The listing builds one solid part. Answer for the finished solid, in the listing's coordinates (mm). A direction names the side the tool comes from. Coordinates: 2 decimals unless noted, no trailing zeros. Loops run counter-clockwise (first coordinate to the right, second up) from the corner with the lowest first, then second, coordinate; pieces in that order, holes last. Notation, with made-up numbers: (81.5, 26) - (138.5, 26) arc R37 ccw to (138.5, 65) - close; hole circle Ø6 at (18, 62). An arc over 180 degrees is marked (long way). Return JSON: item names as keys, results as strings. Group by question number.
1. The mould has two halves that part along Y. Classify faces 1 (the face through (7, 0, 0)), 2 (the face through (-3.47, -15.62, 2.46)), 3 (the face through (10.331, 0.526, 4.341)): pulls with the +Y half, pulls with the -Y half, needs draft (parallel to the pull), parting line crosses it, or undercut.
2. Each of these flat-tipped pins is pushed along its axis until it touches: P1, Ø8, axis at y = -1, z = 17, coming from the +X side; P2, Ø5, axis at x = 12, y = 0, coming from the -Z side; P3, Ø4, axis at x = 8, z = 3.5, coming from the +Y side; P4, Ø2, axis at x = 12, y = 0, coming from the -Z side. Where does it stop, or does it pass through?
3. Section B-B (y = 0) is taken. State how many separate pieces and enclosed holes the cut face has, and give its area (3 significant figures).
4. Section A-A (z = 4.25) is taken. Write down the section's boundary in (x, y), and give its area (3 significant figures).
5. Section D-D (z = 11) is taken. Write down the section's boundary in (x, y).
6. Which of the six approach directions +Z, -Z, +X, -X, +Y, -Y give full straight-line access (tool end or side, diameter ignored) to faces 4 (the face through (0.228, -10.265, 4.341)), 5 (the face through (10.6, -1.4, 3.7)), 6 (the face through (-5.158, -3.955, 24.059))?
7. Find the intervals of material crossed by line 1 along Y through (x, z) = (0, 4.3); line 2 along Y through (x, z) = (0, 13); line 3 along Z through (x, y) = (9.5, -2.5), in increasing order.
```python
from build123d import *

# Parameters (mm, degrees)
IZIM1_R                     = 16
Y_KSEKLIK_EKSTR_ZYON1_DEPTH = 5
IZIM2_R                     = 8
Y_KSEKLIK_EKSTR_ZYON2_DEPTH = 19.7
KES_EKSTR_ZYON1_REACH       = 35.498
IZIM3_R                     = 4
KES_EKSTR_ZYON2_REACH       = 35.498
IZIM4_R                     = 1.75
IZIM4_3_R                   = 3.25
IZIM4_3_R_2                 = 1.75
KES_EKSTR_ZYON3_DEPTH       = 3.7
IZIM5_R                     = 6.5
KES_EKSTR_ZYON4_DEPTH       = 1.3
KES_EKSTR_ZYON5_START       = -23.4
IZIM5_2_R                   = 6.5
KES_EKSTR_ZYON5_DEPTH       = 1.3


with BuildPart() as part:
    # Çizim1 → Yükseklik-Ekstrüzyon1 (new body)
    with BuildSketch(Plane.XY):
        Circle(IZIM1_R)
    extrude(amount=Y_KSEKLIK_EKSTR_ZYON1_DEPTH)

    # Çizim2 → Yükseklik-Ekstrüzyon2 (add)
    with BuildSketch(Plane.XY.offset(5)):
        Circle(IZIM2_R)
    extrude(amount=Y_KSEKLIK_EKSTR_ZYON2_DEPTH)

    # Çizim3 → Kes-Ekstrüzyon1 (cut, up to next)
    with BuildSketch(Plane.XY.offset(24.7), mode=Mode.PRIVATE) as kes_ekstr_zyon1_sk1:
        Circle(IZIM3_R)
    kes_ekstr_zyon1_tool1 = extrude(kes_ekstr_zyon1_sk1.sketch, amount=-KES_EKSTR_ZYON1_REACH, mode=Mode.PRIVATE) & part.part
    add(kes_ekstr_zyon1_tool1.solids().sort_by_distance((0, 0, 24.7))[0], mode=Mode.SUBTRACT)

    # Çizim4 → Kes-Ekstrüzyon2 (cut, up to next)
    with BuildSketch(Plane(origin=(0, 0, 0), x_dir=(-1, 0, 0), z_dir=(0, 0, -1)), mode=Mode.PRIVATE) as kes_ekstr_zyon2_sk1:
        with Locations((0, 12)):
            Circle(IZIM4_R)
    kes_ekstr_zyon2_tool1 = extrude(kes_ekstr_zyon2_sk1.sketch, amount=-KES_EKSTR_ZYON2_REACH, mode=Mode.PRIVATE) & part.part
    # Çizim4 → Kes-Ekstrüzyon2 (cut, up to next)
    with BuildSketch(Plane(origin=(0, 0, 0), x_dir=(-1, 0, 0), z_dir=(0, 0, -1)), mode=Mode.PRIVATE) as kes_ekstr_zyon2_sk2:
        with Locations((12, 0)):
            Circle(IZIM4_R)
    kes_ekstr_zyon2_tool2 = extrude(kes_ekstr_zyon2_sk2.sketch, amount=-KES_EKSTR_ZYON2_REACH, mode=Mode.PRIVATE) & part.part
    # Çizim4 → Kes-Ekstrüzyon2 (cut, up to next)
    with BuildSketch(Plane(origin=(0, 0, 0), x_dir=(-1, 0, 0), z_dir=(0, 0, -1)), mode=Mode.PRIVATE) as kes_ekstr_zyon2_sk3:
        with Locations((0, -12)):
            Circle(IZIM4_R)
    kes_ekstr_zyon2_tool3 = extrude(kes_ekstr_zyon2_sk3.sketch, amount=-KES_EKSTR_ZYON2_REACH, mode=Mode.PRIVATE) & part.part
    # Çizim4 → Kes-Ekstrüzyon2 (cut, up to next)
    with BuildSketch(Plane(origin=(0, 0, 0), x_dir=(-1, 0, 0), z_dir=(0, 0, -1)), mode=Mode.PRIVATE) as kes_ekstr_zyon2_sk4:
        with Locations((-12, 0)):
            Circle(IZIM4_R)
    kes_ekstr_zyon2_tool4 = extrude(kes_ekstr_zyon2_sk4.sketch, amount=-KES_EKSTR_ZYON2_REACH, mode=Mode.PRIVATE) & part.part
    add(kes_ekstr_zyon2_tool1.solids().sort_by_distance((0, 12, 0))[0], mode=Mode.SUBTRACT)
    add(kes_ekstr_zyon2_tool2.solids().sort_by_distance((-12, 0, 0))[0], mode=Mode.SUBTRACT)
    add(kes_ekstr_zyon2_tool3.solids().sort_by_distance((0, -12, 0))[0], mode=Mode.SUBTRACT)
    add(kes_ekstr_zyon2_tool4.solids().sort_by_distance((12, 0, 0))[0], mode=Mode.SUBTRACT)

    # Çizim4<3> → Kes-Ekstrüzyon3 (cut)
    # profile 1 of 4: a face of its own
    with BuildSketch(Plane(origin=(0, 0, 0), x_dir=(-1, 0, 0), z_dir=(0, 0, -1))):
        with Locations((0, 12)):
            Circle(IZIM4_3_R)
        with Locations((0, 12)):
            Circle(IZIM4_3_R_2, mode=Mode.SUBTRACT)
    # profile 2 of 4: a face of its own
    with BuildSketch(Plane(origin=(0, 0, 0), x_dir=(-1, 0, 0), z_dir=(0, 0, -1))):
        with Locations((12, 0)):
            Circle(IZIM4_3_R)
        with Locations((12, 0)):
            Circle(IZIM4_3_R_2, mode=Mode.SUBTRACT)
    # profile 3 of 4: a face of its own
    with BuildSketch(Plane(origin=(0, 0, 0), x_dir=(-1, 0, 0), z_dir=(0, 0, -1))):
        with Locations((0, -12)):
            Circle(IZIM4_3_R)
        with Locations((0, -12)):
            Circle(IZIM4_3_R_2, mode=Mode.SUBTRACT)
    # profile 4 of 4: a face of its own
    with BuildSketch(Plane(origin=(0, 0, 0), x_dir=(-1, 0, 0), z_dir=(0, 0, -1))):
        with Locations((-12, 0)):
            Circle(IZIM4_3_R)
        with Locations((-12, 0)):
            Circle(IZIM4_3_R_2, mode=Mode.SUBTRACT)
    extrude(amount=-KES_EKSTR_ZYON3_DEPTH, mode=Mode.SUBTRACT)

    # Çizim5 → Kes-Ekstrüzyon4 (cut)
    with BuildSketch(Plane.XY.offset(24.7)):
        Circle(IZIM5_R)
    extrude(amount=-KES_EKSTR_ZYON4_DEPTH, mode=Mode.SUBTRACT)

    # Çizim5<2> → Kes-Ekstrüzyon5 (cut)
    with BuildSketch(Plane.XY.offset(24.7).offset(KES_EKSTR_ZYON5_START)):
        Circle(IZIM5_2_R)
    extrude(amount=-KES_EKSTR_ZYON5_DEPTH, mode=Mode.SUBTRACT)


solid = part.part
```
The answers:
{
 "1": {"face 1": "needs draft", "face 2": "parting line crosses it", "face 3": "undercut"},
 "2": {"P1": "stops at x = 8", "P2": "stops at z = 3.7", "P3": "stops at y = 14.83", "P4": "passes through"},
 "3": {"separate pieces": "4", "enclosed holes": "0", "area": "207 mm2"},
 "4": {"outline": "circle Ø32 at (0, 0); hole circle Ø3.5 at (-12, 0); hole circle Ø8 at (0, 0); hole circle Ø3.5 at (0, -12); hole circle Ø3.5 at (0, 12); hole circle Ø3.5 at (12, 0)", "area": "715 mm2"},
 "5": {"outline": "circle Ø16 at (0, 0); hole circle Ø8 at (0, 0)"},
 "6": {"face 4": "+Z, -Z", "face 5": "-Z", "face 6": "+Z"},
 "7": {"line 1": "y = -16 to -13.75, -10.25 to -4, 4 to 10.25, 13.75 to 16", "line 2": "y = -8 to -4, 4 to 8", "line 3": "z = 0 to 5"}
}
